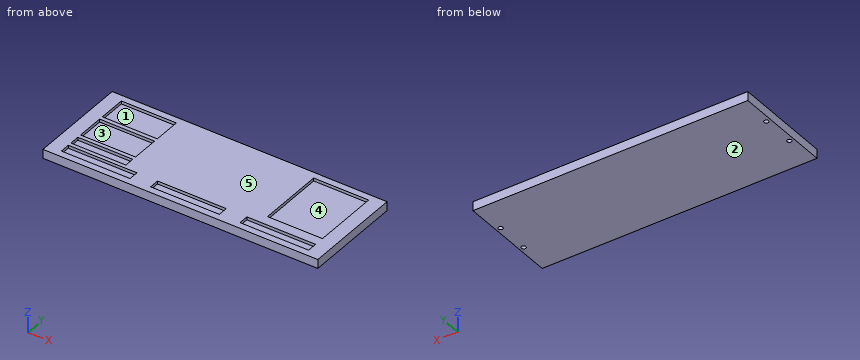
Autodesk Inventor part; units mm, degrees
ref_plane "YZ Plane" through (0, 0, 0) normal (1, 0, 0) x (0, 1, 0)
ref_plane "XZ Plane" through (0, 0, 0) normal (0, 1, 0) x (-1, 0, 0)
ref_plane "XY Plane" through (0, 0, 0) normal (0, 0, 1) x (1, 0, 0)
sketch "Boceto1" plane through (0, 0, 0) normal (0, 0, 1) x (1, 0, 0)
  line L0 (-275, -100) -> (275, -100)
  line L1 (275, -100) -> (275, 100)
  line L2 (275, 100) -> (-275, 100)
  line L3 (-275, 100) -> (-275, -100)
  line L4 (-275, -100) -> (275, 100) construction
  line L5 (275, -100) -> (-275, 100) construction
  point P0 (0, 0)
  dimension "ancho" = 550
  dimension "alto" = 200
extrude "Extrusión1" add sketch "Boceto1" along normal blind 18
sketch "Boceto2" plane through (0, 0, 18) normal (0, 0, 1) x (1, 0, 0)
  line L0 (247.5, -86.6667) -> (110, -86.6667)
  line L1 (110, -86.6667) -> (110, -66.6667)
  line L2 (110, -66.6667) -> (247.5, -66.6667)
  line L3 (247.5, -66.6667) -> (247.5, -86.6667)
  line L4 (275, -100) -> (275, 100)
  line L5 (-110, -86.6667) -> (-247.5, -86.6667)
  line L6 (-247.5, -86.6667) -> (-247.5, -66.6667)
  line L7 (-247.5, -66.6667) -> (-110, -66.6667)
  line L8 (-110, -66.6667) -> (-110, -86.6667)
  line L9 (-275, 100) -> (-275, -100)
  line L10 (-275, -100) -> (275, -100)
  line L11 (68.75, -86.6667) -> (-68.75, -86.6667)
  line L12 (-68.75, -86.6667) -> (-68.75, -66.6667)
  line L13 (-68.75, -66.6667) -> (68.75, -66.6667)
  line L14 (68.75, -66.6667) -> (68.75, -86.6667)
  line L15 (275, 100) -> (-275, 100)
  line L16 (247.5, 86.6667) -> (137.5, 86.6667)
  line L17 (137.5, 86.6667) -> (137.5, -46.6667)
  line L18 (137.5, -46.6667) -> (247.5, -46.6667)
  line L19 (247.5, -46.6667) -> (247.5, 86.6667)
  line L20 (-247.5, 86.6667) -> (-137.5, 86.6667)
  line L21 (-137.5, 86.6667) -> (-137.5, 31.6667)
  line L22 (-137.5, 31.6667) -> (-247.5, 31.6667)
  line L23 (-247.5, 31.6667) -> (-247.5, 86.6667)
  line L24 (-247.5, 23.8235) -> (-137.5, 23.8235)
  line L25 (-137.5, 23.8235) -> (-137.5, -31.1765)
  line L26 (-137.5, -31.1765) -> (-247.5, -31.1765)
  line L27 (-247.5, -31.1765) -> (-247.5, 23.8235)
  line L28 (-247.5, -59.0196) -> (-137.5, -59.0196)
  line L29 (-137.5, -59.0196) -> (-137.5, -39.0196)
  line L30 (-137.5, -39.0196) -> (-247.5, -39.0196)
  line L31 (-247.5, -39.0196) -> (-247.5, -59.0196)
  point P0 (0, 0)
  dimension "d4" = 137.5
  dimension "d5" = 20
  dimension "d6" = 27.5
  dimension "d7" = 137.5
  dimension "d8" = 20
  dimension "d9" = 27.5
  dimension "d10" = 13.3333
  dimension "d11" = 13.3333
  dimension "d12" = 137.5
  dimension "d13" = 41.25
  dimension "d14" = 41.25
  dimension "d15" = 20
  dimension "d17" = 110
  dimension "d18" = 133.3333
  dimension "d19" = 27.5
  dimension "d20" = 13.3333
  dimension "d21" = 110
  dimension "d22" = 55
  dimension "d23" = 27.5
  dimension "d24" = 13.3333
  dimension "d25" = 110
  dimension "d26" = 55
  dimension "d27" = 27.5
  dimension "d28" = 7.8431
  dimension "d29" = 110
  dimension "d30" = 20
  dimension "d31" = 7.8431
  dimension "d32" = 7.6471
extrude "Extrusión2" cut sketch "Boceto2" against normal blind 6 contours L0 L1 L2 L3 | L5 L6 L7 L8 | L11 L12 L13 L14 | L19 L18 L17 L16 | L20 L21 L22 L23 | L24 L25 L26 L27 | L31 L30 L29 L28
sketch "Boceto3" plane through (0, 0, 0) normal (0, 0, -1) x (-1, 0, 0)
  circle A0 centre (266, -33.3333) radius 4.5
  circle A1 centre (266, 33.3333) radius 4.5
  circle A2 centre (-266, 33.3333) radius 4.5
  circle A3 centre (-266, -33.3333) radius 4.5
  line L0 (275, 100) -> (275, -100)
  line L1 (275, -100) -> (-275, -100)
  line L2 (-275, 100) -> (275, 100)
  line L3 (-275, -100) -> (-275, 100)
  point P0 (0, 0)
  dimension "d35" = 9
  dimension "d36" = 9
  dimension "d37" = 9
  dimension "d38" = 9
  dimension "d39" = 9
  dimension "d40" = 66.6667
  dimension "d41" = 9
  dimension "d42" = 66.6667
  dimension "d43" = 9
  dimension "d44" = 66.6667
  dimension "d45" = 9
  dimension "d46" = 66.6667
extrude "Extrusión3" cut sketch "Boceto3" against normal blind 6 contours A0 | A1 | A2 | A3
equation "\"d4\" = 0.25 * ancho"
equation "\"d5\" = 0.1 * alto"
equation "\"d6\" = 0.05 * ancho"
equation "\"d7\" = d4"
equation "\"d8\" = d5"
equation "\"d9\" = d6"
equation "\"d10\" = 0.0666667 * alto"
equation "\"d11\" = 0.0666667 * alto"
equation "\"d12\" = d4"
equation "\"d13\" = d14"
equation "\"d15\" = d5"
equation "\"d17\" = 0.2 * ancho"
equation "\"d18\" = 0.666667 * alto"
equation "\"d19\" = d6"
equation "\"d20\" = d10"
equation "\"d21\" = 0.2 * ancho"
equation "\"d22\" = 0.1 * ancho"
equation "\"d23\" = d9"
equation "\"d24\" = d11"
equation "\"d25\" = d21"
equation "\"d26\" = d22"
equation "\"d27\" = d23"
equation "\"d28\" = 0.0392157 * alto"
equation "\"d29\" = d21"
equation "\"d30\" = d5"
equation "\"d31\" = d28"
equation "\"d33\" = 0.333333 * grosor"
equation "\"d35\" = 0.5 * grosor"
equation "\"d36\" = d35"
equation "\"d37\" = d35"
equation "\"d38\" = d35"
equation "\"d39\" = 0.5 * grosor"
equation "\"d40\" = 0.333333 * alto"
equation "\"d41\" = d39"
equation "\"d42\" = d40"
equation "\"d43\" = d39"
equation "\"d44\" = d40"
equation "\"d45\" = d39"
equation "\"d46\" = d40"
equation "\"d47\" = 0.333333 * grosor"
properties part number "Base"
Build history of the part. All positions in model axes, mm. Face numbers are marked on the shaded views. A direction names the side the tool comes from. Give positions to 0.01 mm unless a question says otherwise; leave off trailing zeros. Loops run counter-clockwise (first coordinate to the right, second up) from the corner with the lowest first, then second, coordinate; pieces in that order, holes last.
Item 1: Pull direction Y, two halves, no side cores. Call the marked faces 3, 4 and 5: released by +Y, released by -Y, zero draft, split by the parting line, or undercut.
Answers follow:
face 3: undercut
face 4: undercut
face 5: zero draft
Item 2: Flat gauge pins, fed straight in: pin 1 (7 mm diameter, centred on x = -266, y = -33.33, fed in from -Z); pin 2 (5 mm diameter, centred on x = -161, y = 67, fed in from +Z). Where does each tip first touch, or does it go through?
Answers follow:
pin 1: stops at z = 6
pin 2: stops at z = 12
Item 3: Slice it at B-B, the plane y = 1. List the corners of the cut face in (x, z), and give its area (3 significant figures).
Answers follow:
outline: (-275, 0) - (275, 0) - (275, 18) - (247.5, 18) - (247.5, 12) - (137.5, 12) - (137.5, 18) - (-137.5, 18) - (-137.5, 12) - (-247.5, 12) - (-247.5, 18) - (-275, 18) - close
area: 8,580 mm2
Item 4: Slice it at D-D, the plane y = -78. List the corners of the cut face in (x, z).
Answers follow:
outline: (-275, 0) - (275, 0) - (275, 18) - (247.5, 18) - (247.5, 12) - (110, 12) - (110, 18) - (68.75, 18) - (68.75, 12) - (-68.75, 12) - (-68.75, 18) - (-110, 18) - (-110, 12) - (-247.5, 12) - (-247.5, 18) - (-275, 18) - close
Item 5: Slice it at A-A, the plane x = -24. List the corners of the cut face in (y, z), and give its area (3 significant figures).
Answers follow:
outline: (-100, 0) - (100, 0) - (100, 18) - (-66.67, 18) - (-66.67, 12) - (-86.67, 12) - (-86.67, 18) - (-100, 18) - close
area: 3,480 mm2
Item 6: Drill centre lines: line 1 (Y direction, x = 266, z = 1.4); line 2 (Y direction, x = -223, z = 14.75); line 3 (X direction, y = 15, z = 14.75). Where is each one in solid material? Low to high.
Answers follow:
line 1: y = -100 to -37.83, -28.83 to 28.83, 37.83 to 100
line 2: y = -100 to -86.67, -66.67 to -59.02, -39.02 to -31.18, 23.82 to 31.67, 86.67 to 100
line 3: x = -275 to -247.5, -137.5 to 137.5, 247.5 to 275
Item 7: Which spindle directions (+Z, -Z, +X, -X, +Y, -Y) get a long thin tool onto all of the face, cutting with end or side? Do the marked faces 1 and 2. Say none if no direction does.
Answers follow:
face 1: +Z
face 2: -Z, +X, -X, +Y, -Y
Item 8: Slice it at C-C, the plane x = -175. List the corners of the cut face in (y, z), and give its area (3 significant figures).
Answers follow:
outline: (-100, 0) - (100, 0) - (100, 18) - (86.67, 18) - (86.67, 12) - (31.67, 12) - (31.67, 18) - (23.82, 18) - (23.82, 12) - (-31.18, 12) - (-31.18, 18) - (-39.02, 18) - (-39.02, 12) - (-59.02, 12) - (-59.02, 18) - (-66.67, 18) - (-66.67, 12) - (-86.67, 12) - (-86.67, 18) - (-100, 18) - close
area: 2,700 mm2
